Design review of the part shown in the three views and the two pictorial views. Dimensions are in mm from the part's minimum x, y and z. Give positions to 0.01 mm unless a question says otherwise; leave off trailing zeros. Loops run counter-clockwise (first coordinate to the right, second up) from the corner with the lowest first, then second, coordinate; pieces in that order, holes last. Notation, with made-up numbers: (16.25, 3) -> (23.25, 3) arc R10 ccw to (23.25, 16) -> close; hole circle Ø11 at (11, 81.5). An arc over 180 degrees is marked (long way). Answer as CSV lines item,"result".
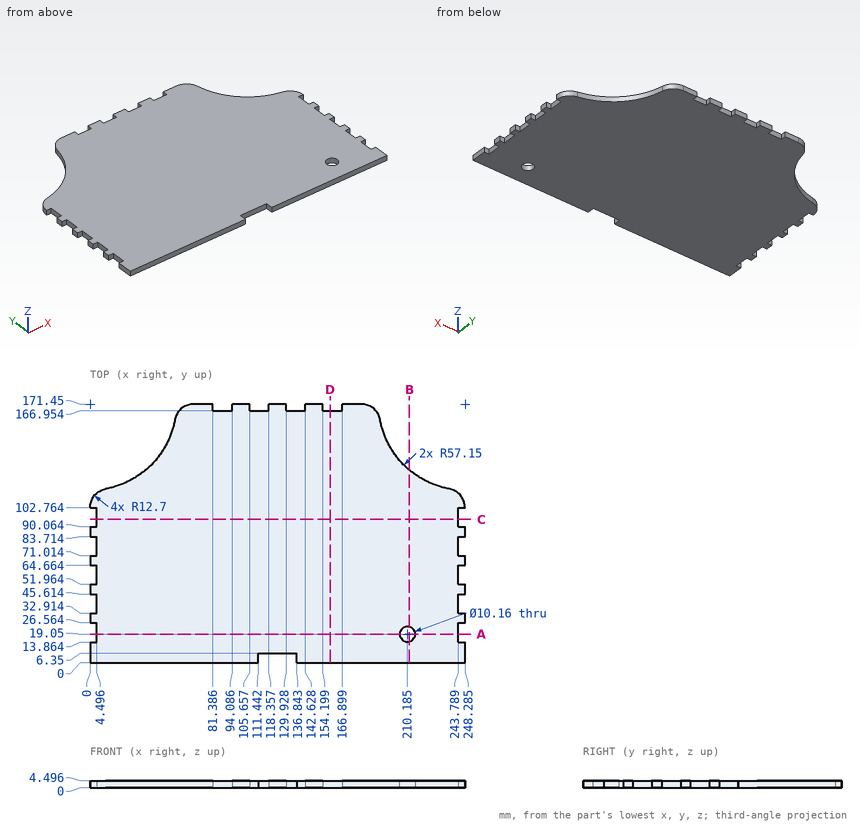
Q1. We need section D-D, the plane x = 159. State the section outline as (y, z) points (1 decimal).
Filled sheet:
outline,"(0, 0) -> (167, 0) -> (167, 4.5) -> (0, 4.5) -> close"
Q2. To check wall thickness, follow probe 1 along Y at (x, z) = (108, 1.75) (1 decimal); probe 2 along X at (y, z) = (59, 1.15) (1 decimal); probe 3 along Y at (x, z) = (60, 1.45) (1 decimal). State the ranges of each line that lie inside material, in increasing order. Write a range as from..to.
Filled sheet:
probe 1,"y = 0..167"
probe 2,"x = 4.5..243.8"
probe 3,"y = 0..168"
Q3. We need section A-A, the plane y = 19.05. State the section outline as (x, z) points (1 decimal), and give its area (3 significant figures).
Filled sheet:
outline,"(4.5, 0) -> (205.1, 0) -> (205.1, 4.5) -> (4.5, 4.5) -> close; (215.3, 0) -> (243.8, 0) -> (243.8, 4.5) -> (215.3, 4.5) -> close"
area,"1,030 mm^2"
Q4. We need section B-B, the plane x = 211.5. State the section outline as (y, z) points (1 decimal), and give its area (3 significant figures).
Filled sheet:
outline,"(0, 0) -> (14.1, 0) -> (14.1, 4.5) -> (0, 4.5) -> close; (24, 0) -> (127.7, 0) -> (127.7, 4.5) -> (24, 4.5) -> close"
area,"530 mm^2"
Q5. We need section C-C, the plane y = 95. State the section outline as (x, z) points (1 decimal).
Filled sheet:
outline,"(4.5, 0) -> (243.8, 0) -> (243.8, 4.5) -> (4.5, 4.5) -> close"
Q6. Clearance check with flat-ended pins moving along their axes: pin 1 Ø1.3 at (x, z) = (3, 1.5) entering from +Y (1 decimal); pin 2 Ø1.3 at (y, z) = (170, 3.5) entering from +X (1 decimal); pin 3 Ø1.3 at (x, z) = (110, 1) entering from +Y. State where each tip first meets the part, or that it passes through.
Filled sheet:
pin 1,"stops at y = 111.7"
pin 2,"stops at x = 186.6"
pin 3,"stops at y = 166.95"
